CAD build for the part. Positions are in the model's coordinates, mm. A direction names the side the tool comes from. Give positions to 0.01 mm unless a question says otherwise; leave off trailing zeros. Loops run counter-clockwise (first coordinate to the right, second up) from the corner with the lowest first, then second, coordinate; pieces in that order, holes last.
```python
from build123d import *

# Parameters (mm, degrees)
F0_W     = 85
F0_H     = 15
F1_DEPTH = 5
F2_W     = 34
F2_H     = 2
F3_DEPTH = 5.001


with BuildPart() as f1:
    # F0 (on Top) → F1 (new body)
    with BuildSketch(Plane.XY):
        Rectangle(F0_W, F0_H)
    extrude(amount=F1_DEPTH)

    # F2 (on Top) → F3 (cut, through all)
    with BuildSketch(Plane.XY):
        with Locations((-22.451008, 3.5)):
            Rectangle(F2_W, F2_H)
        with Locations((22.451008, 3.5)):
            Rectangle(F2_W, F2_H)
    extrude(amount=F3_DEPTH, mode=Mode.SUBTRACT)


solid = f1.part
```
1. Pull direction Y, two halves, no side cores. Call faces 3 (the face through (-1, 7.5, 2)), 4 (the face through (-42.5, 0, 2)), 5 (the face through (-23, 2.5, 2)): released by +Y, released by -Y, zero draft, split by the parting line, or undercut.
Responses:
face 3: released by +Y
face 4: zero draft
face 5: undercut
2. Saw through at A-A, the plane y = 3.75. List the corners of the cut face in (x, z), and give its area (3 significant figures).
Responses:
outline: (-42.5, 0) - (-39.45, 0) - (-39.45, 5) - (-42.5, 5) - close; (-5.45, 0) - (5.45, 0) - (5.45, 5) - (-5.45, 5) - close; (39.45, 0) - (42.5, 0) - (42.5, 5) - (39.45, 5) - close
area: 85.0 mm2
3. Probe line 1 along Y through (x, z) = (31, 0.6). List the from-to ranges inside material, lowest first.
Responses:
line 1: y = -7.5 to 2.5, 4.5 to 7.5
4. Saw through at B-B, the plane x = 10. List the corners of the cut face in (y, z).
Responses:
outline: (-7.5, 0) - (2.5, 0) - (2.5, 5) - (-7.5, 5) - close; (4.5, 0) - (7.5, 0) - (7.5, 5) - (4.5, 5) - close
5. Tool access for faces 1 (the face through (22, 4.5, 2)), 2 (the face through (42.5, 0, 2)): list every direction of +Z, -Z, +X, -X, +Y, -Y with a clear straight run to the whole face (end or side of a thin tool).
Responses:
face 1: +Z, -Z
face 2: +Z, -Z, +X, +Y, -Y
6. Saw through at C-C, the plane z = 2.2. List the corners of the cut face in (x, y), and give its area (3 significant figures).
Responses:
outline: (-42.5, -7.5) - (42.5, -7.5) - (42.5, 7.5) - (-42.5, 7.5) - close; hole (-39.45, 2.5) - (-5.45, 2.5) - (-5.45, 4.5) - (-39.45, 4.5) - close; hole (5.45, 2.5) - (39.45, 2.5) - (39.45, 4.5) - (5.45, 4.5) - close
area: 1,140 mm2
